from build123d import *

# Parameters (mm, degrees)
BASE_EXTRUDE_DEPTH              = 8
BOSS_EXTRUDE1_DEPTH             = 73
BOSS_EXTRUDE3_DEPTH             = 8
F_8_0_DIAMETER_HOLE1_D          = 8
F_8_32_TAPPED_HOLE1_D           = 3.4544
F_8_32_TAPPED_HOLE1_DEPTH       = 12.2936
F_8_32_TAPPED_HOLE1_CBORE_D     = 4.1656
F_8_32_TAPPED_HOLE1_CBORE_DEPTH = 8.3312
F_8_32_TAPPED_HOLE1_TIP         = 1.037806461
F_10_32_TAPPED_HOLE1_D          = 4.826
CUT_EXTRUDE1_DEPTH              = 3.5
HOLE1_D                         = 4
HOLE1_DEPTH                     = 3.5
SKETCH14_W                      = 12.1518
SKETCH14_H                      = 18.1
BOSS_EXTRUDE2_DEPTH             = 16.5
CHAMFER1_SIZE                   = 1


with BuildPart() as part:
    # Sketch1 → Base-Extrude (new body)
    with BuildSketch(Plane.XY.offset(-1048.957398403)):
        Polygon((-6.1741, 23), (23.3259, 23), (23.3259, 10.2), (23.1259, 10), (23.1259, -10), (23.3259, -10.2), (23.3259, -23), (-6.1741, -23), align=None)
    extrude(amount=BASE_EXTRUDE_DEPTH)

    # Sketch3 → Boss-Extrude1 (add)
    with BuildSketch(Plane(origin=(0, 0, -1048.957398403), x_dir=(-1, 0, 0), z_dir=(0, 0, -1))):
        Polygon((-23.3259, 10.2), (-23.3259, 23), (-8.6741, 23), (-8.6741, -23), (-23.3259, -23), (-23.3259, -10.2), (-23.1259, -10), (-23.1259, 10), align=None)
    extrude(amount=BOSS_EXTRUDE1_DEPTH)

    # Sketch15 → Boss-Extrude3 (add)
    with BuildSketch(Plane.XY.offset(-1040.957398403)):
        Polygon((23.1259, -10), (23.1259, 10), (23.3259, 10.2), (23.3259, -10.2), align=None)
    extrude(amount=-BOSS_EXTRUDE3_DEPTH)

    # 8.0 Diameter Hole1 (through all)
    with Locations(Plane(origin=(23.1259, 0, 0), x_dir=(0, 0, -1), z_dir=(1, 0, 0))):
        with Locations((1073.957398403, 0)):
            Hole(F_8_0_DIAMETER_HOLE1_D / 2)

    # #8-32 Tapped Hole1
    with Locations(Plane(origin=(23.3259, 0, 0), x_dir=(0, 0, -1), z_dir=(1, 0, 0))):
        with Locations((1056.957398403, 14), (1091.957398403, 14), (1056.957398403, -14), (1091.957398403, -14)):
            CounterBoreHole(F_8_32_TAPPED_HOLE1_D / 2, F_8_32_TAPPED_HOLE1_CBORE_D / 2, F_8_32_TAPPED_HOLE1_CBORE_DEPTH, depth=F_8_32_TAPPED_HOLE1_DEPTH)
            with Locations((0, 0, -(F_8_32_TAPPED_HOLE1_DEPTH + F_8_32_TAPPED_HOLE1_TIP / 2))):  # 118° drill point
                Cone(0, F_8_32_TAPPED_HOLE1_D / 2, F_8_32_TAPPED_HOLE1_TIP, mode=Mode.SUBTRACT)

    # #10-32 Tapped Hole1 (through all)
    with Locations(Plane.XY.offset(-1040.957398403)):
        with Locations((7.3259, 19), (7.3259, -19)):
            Hole(F_10_32_TAPPED_HOLE1_D / 2)

    # Sketch11 → Cut-Extrude1 (cut)
    with BuildSketch(Plane(origin=(23.1259, 0, 0), x_dir=(0, 0, -1), z_dir=(1, 0, 0))):
        with BuildLine():
            Line((1091.457398403, 2), (1092.457398403, 2))
            ThreePointArc((1092.457398403, 2), (1094.457398403, 0), (1092.457398403, -2))
            Line((1092.457398403, -2), (1091.457398403, -2))
            ThreePointArc((1091.457398403, -2), (1089.457398403, 0), (1091.457398403, 2))
        make_face()
    extrude(amount=-CUT_EXTRUDE1_DEPTH, mode=Mode.SUBTRACT)

    # Hole1
    with Locations(Plane(origin=(23.1259, 0, 0), x_dir=(0, 0, -1), z_dir=(1, 0, 0))):
        with Locations((1056.957398403, 0)):
            Hole(HOLE1_D / 2, depth=HOLE1_DEPTH)

    # Sketch14 → Boss-Extrude2 (add)
    with BuildSketch(Plane(origin=(0, 23, 0), x_dir=(-1, 0, 0), z_dir=(0, 1, 0))):
        with Locations((-15.75, -1080.007398403)):
            Rectangle(SKETCH14_W, SKETCH14_H)
    extrude(amount=BOSS_EXTRUDE2_DEPTH)

    # Chamfer1
    chamfer1_edges = [part.edges().sort_by_distance(p)[0] for p in [
        (23.3259, -23, -1081.457398403),
        (23.3259, 23, -1081.457398403),
    ]]
    chamfer(chamfer1_edges, length=CHAMFER1_SIZE)


solid = part.part
Here's how the part is built. I have some questions about the finished solid (model axes, mm). A direction names the side the tool comes from. Coordinates: 2 decimals unless noted, no trailing zeros. Order: outer loops, then holes, each group sorted by start corner. A loop starts at its lowest first (then second) coordinate and runs counter-clockwise, first axis right, second up. Notation, with made-up numbers: (54.25, 51.5) - (113.25, 51.5) arc R26 cw to (113.25, 90.5) - close; hole circle Ø3 at (38, 33.5). An arc over 180 degrees is marked (long way). Use CSV: the item, a comma, the result in double quotes. Start each with the question number.
1. I'm going to push flat-ended pins straight in: pin 1 (12 mm diameter, centred on x = 20, y = 27, fed in from +Z); pin 2 (3 mm diameter, centred on y = 14, z = -1056.96, fed in from -X); pin 3 (10 mm diameter, centred on y = 0.5, z = -1082.5, fed in from +X); pin 4 (9.5 mm diameter, centred on x = 19, y = 28, fed in from -Z). Where does each tip first touch, or does it pass through?
2. Please list where these lines run through material, in increasing order: line 1 (Z direction, x = 13, y = 14); line 2 (Y direction, x = 15.75, z = -1074); line 3 (X direction, y = -19.5, z = -1075). Write a range as from..to.
3. Suppose I cut it at D-D on y = 0. List the corners of the cut face in (x, z) for me, then the cut area to 3 significant figures.
4. For faces 1 (the face through (19.219, -13.374, -1058.944)), 2 (the face through (9.674, 31, -1080)), 3 (the face through (9.737, 19.106, -1073.024)), 4 (the face through (23.126, 0, -1085)), which set-ups out of +Z, -Z, +X, -X, +Y, -Y let a thin tool reach every point of the face, with its end or its side?
5. Suppose I cut it at B-B on x = 17. List the corners of the cut face in (y, z) for me, then the cut area to 3 significant figures.
6. If we mould it in two halves opening along Z, with no side actions, what happens to faces 5 (the face through (13, 15.2, -1058.2)), 6 (the face through (16, 31, -1070.957)), 7 (the face through (9.737, -18.894, -1073.024))? For each: +Z half, -Z half, draft (parallel to the pull), parting line (faces both ways), or undercut.
7. Suppose I cut it at C-C on z = -1108. List the corners of the cut face in (x, y) for me, then the cut area to 3 significant figures.
8. Suppose I cut it at A-A on y = 19. List the corners of the cut face in (x, z) for me, then the cut area to 3 significant figures.
Output:
1,pin 1,"stops at z = -1040.96"
1,pin 2,"stops at x = 8.67"
1,pin 3,"stops at x = 23.13"
1,pin 4,"stops at z = -1089.06"
2,line 1,"z = -1121.96..-1093.68, -1090.23..-1058.68, -1055.23..-1040.96"
2,line 2,"y = -23..-4, 4..39.5"
2,line 3,"x = 9.69..23.33"
3,outline,"(-6.17, -1048.96) - (8.67, -1048.96) - (8.67, -1069.96) - (23.13, -1069.96) - (23.13, -1058.96) - (19.63, -1058.96) - (19.63, -1054.96) - (23.13, -1054.96) - (23.13, -1048.96) - (23.33, -1048.96) - (23.33, -1040.96) - (-6.17, -1040.96) - close; (8.67, -1121.96) - (23.13, -1121.96) - (23.13, -1094.46) - (19.63, -1094.46) - (19.63, -1089.46) - (23.13, -1089.46) - (23.13, -1077.96) - (8.67, -1077.96) - close"
3,area,"1,140 mm2"
4,face 1,"+X"
4,face 2,"+Z, -Z, -X, +Y"
4,face 3,"+Z, -Z"
4,face 4,"-Z, +X"
5,outline,"(-23, -1121.96) - (23, -1121.96) - (23, -1089.06) - (39.5, -1089.06) - (39.5, -1070.96) - (23, -1070.96) - (23, -1040.96) - (-23, -1040.96) - close; hole circle Ø4.17 at (-14, -1091.96); hole circle Ø4.17 at (-14, -1056.96); hole circle Ø8 at (0, -1073.96); hole circle Ø4.17 at (14, -1091.96); hole circle Ø4.17 at (14, -1056.96)"
5,area,"3,920 mm2"
6,face 5,"undercut"
6,face 6,"+Z half"
6,face 7,"draft"
7,outline,"(8.67, -23) - (22.33, -23) - (23.33, -22) - (23.33, -10.2) - (23.13, -10) - (23.13, 10) - (23.33, 10.2) - (23.33, 22) - (22.33, 23) - (8.67, 23) - (8.67, 21) arc R2.41 cw to (8.67, 17) - (8.67, -17) arc R2.41 cw to (8.67, -21) - close"
7,area,"663 mm2"
8,outline,"(-6.17, -1048.96) - (4.91, -1048.96) - (4.91, -1040.96) - (-6.17, -1040.96) - close; (9.74, -1121.96) - (23.33, -1121.96) - (23.33, -1040.96) - (9.74, -1040.96) - close"
8,area,"1,190 mm2"
